Design review of the part built by this model. Coordinates are the model's own, in mm. Face numbers are marked on the shaded views. A direction names the side the tool comes from. Coordinates: 2 decimals unless noted, no trailing zeros. Order: outer loops, then holes, each group sorted by start corner. A loop starts at its lowest first (then second) coordinate and runs counter-clockwise, first axis right, second up. Notation, with made-up numbers: (31.25, -14) - (54.25, -14) arc R20 ccw to (54.25, 12) - close; hole circle Ø4 at (12, 62.25). An arc over 180 degrees is marked (long way). Write item = value, one per line. Start each with the question number.
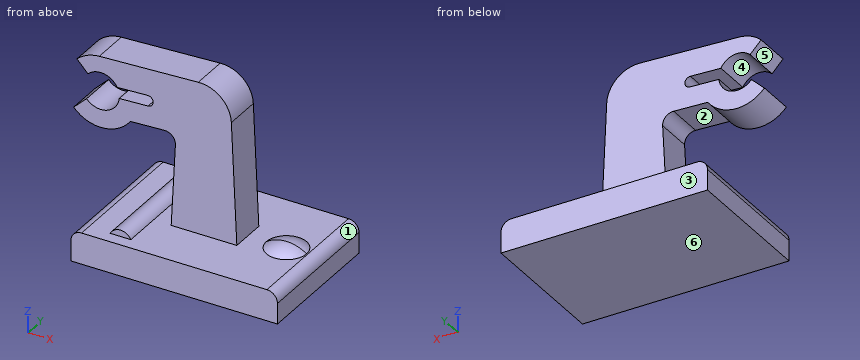
```python
from build123d import *

# Parameters (mm, degrees)
PAD_DEPTH        = 6.5
PAD001_DEPTH     = 5.35
REVOLUTION_ANGLE = -180
PAD002_DEPTH     = 1.75


with BuildPart() as part:
    # Sketch → Pad (new body)
    with BuildSketch(Plane.XZ):
        with BuildLine():
            Line((-9.75, 0), (9.75, 0))
            Line((9.75, 0), (9.75, 1.95))
            ThreePointArc((9.75, 1.95), (9.457107, 2.657107), (8.75, 2.95))
            Line((8.75, 2.95), (-8.75, 2.95))
            ThreePointArc((-8.75, 2.95), (-9.457107, 2.657107), (-9.75, 1.95))
            Line((-9.75, 1.95), (-9.75, 0))
        make_face()
    pad = extrude(amount=-PAD_DEPTH)

    # Sketch001 → Pad001 (join)
    with BuildSketch(Plane.XZ):
        with BuildLine():
            ThreePointArc((-4.775, 2.95), (-5.75, 3.55), (-6.725, 2.95))
            Line((-6.725, 2.95), (-4.775, 2.95))
        make_face()
    pad001 = extrude(amount=-PAD001_DEPTH)

    # Sketch002 → Revolution (revolve)
    with BuildSketch(Plane.XZ):
        with BuildLine():
            ThreePointArc((8.65, 2.95), (7.746243, 3.396436), (6.75, 3.55))
            Line((6.75, 3.55), (6.75, 0.241667))
            Line((8.65, 2.95), (6.75, 0.241667))
        make_face()
    revolution = revolve(axis=Axis((6.75, 0, 3.55), (0, 0, -1)), revolution_arc=REVOLUTION_ANGLE)

    # Sketch003 → Pad002 (join)
    with BuildSketch(Plane.XZ):
        with BuildLine():
            Line((-3.1, 2.95), (3.1, 2.95))
            Line((3.1, 2.95), (2.580696, 14.438223))
            ThreePointArc((2.580696, 14.438223), (1.609703, 16.515339), (-0.544721, 17.3))
            Line((-0.544721, 17.3), (-9.889288, 16.899445))
            ThreePointArc((-9.889288, 16.899445), (-11.025908, 16.641713), (-11.998693, 15.999824))
            Line((-11.998693, 15.999824), (-10.959931, 14.914345))
            ThreePointArc((-8.203688, 14.469402), (-9.471106, 15.377634), (-10.959931, 14.914345))
            Line((-8.203688, 14.469402), (-5.32558, 14.592772))
            ThreePointArc((-5.282715, 13.592772), (-4.804147, 14.114205), (-5.32558, 14.592772))
            Line((-5.282715, 13.592772), (-8.008679, 13.475924))
            ThreePointArc((-11.081461, 12.514345), (-9.227358, 11.979867), (-8.008679, 13.475924))
            Line((-12.311103, 11.337624), (-11.081461, 12.514345))
            ThreePointArc((-12.311103, 11.337624), (-9.56498, 10.204409), (-6.956, 11.62518))
            Line((-3.742396, 11.762931), (-6.956, 11.62518))
            ThreePointArc((-2.700889, 10.712502), (-2.989454, 11.467933), (-3.742396, 11.762931))
            Line((-3.1, 2.95), (-2.700889, 10.712502))
        make_face()
    pad002 = extrude(amount=-PAD002_DEPTH)

    # Mirrored: Pad, Pad001, Revolution, Pad002 across XZ
    add(pad.mirror(Plane.XZ))
    add(pad001.mirror(Plane.XZ))
    add(revolution.mirror(Plane.XZ))
    add(pad002.mirror(Plane.XZ))


solid = part.part
```
Item 1: Add section C-C on z = 1. Give the boundary of the cut face in (x, y).
Item 2: Add section B-B on x = -1.5. Give the boundary of the cut face in (y, z).
Item 3: For line 1 (Z direction, x = -8.25, y = 1.5); line 2 (X direction, y = -3.25, z = 2); line 3 (Z direction, x = -4, y = -3), list the stretches that pass through material, from the lowest coordinate up.
Item 4: Add section D-D on x = 3.75. Give the boundary of the cut face in (y, z).
Item 5: For the marked faces 4, 5 and 6, list the 3-axis set-ups (+Z, -Z, +X, -X, +Y, -Y) from which the entire face can be reached by the end or side of a thin tool; tool diameter is ignored.
Item 6: Mouldability with a two-part tool opening along X and no side actions: class the marked faces 1, 2 and 3 as +X half, -X half, draft (parallel to the pull), parting line (faces both ways), or undercut.
Item 7: Add section A-A on y = 3.25. Give the boundary of the cut face in (x, z) (3 decimals), plus the area to 3 significant figures.
Item 8: For P1, Ø6, axis at x = -3.5, y = -1, coming from the +Z side; P2, Ø5, axis at x = -4.5, z = 15.5, coming from the +Y side; P3, Ø4, axis at y = -3.5, z = 5, coming from the -X side; P4, Ø1, axis at y = -1, z = 1, coming from the -X side, all flat-tipped, find the tip position at first contact; note any pin that passes through.
Worked out:
q1.outline = (-9.75, -6.5) - (9.75, -6.5) - (9.75, 6.5) - (-9.75, 6.5) - close
q2.outline = (-6.5, 0) - (6.5, 0) - (6.5, 2.95) - (1.75, 2.95) - (1.75, 17.26) - (-1.75, 17.26) - (-1.75, 2.95) - (-6.5, 2.95) - close
q3.line_1 = 0 to 2.95, 10.54 to 12.75, 14.55 to 16.97
q3.line_2 = -9.75 to 9.75
q3.line_3 = 0 to 2.95
q4.outline = (-6.5, 0) - (6.5, 0) - (6.5, 2.95) - (-6.5, 2.95) - close
q5.face_4 = +Y, -Y
q5.face_5 = -X, +Y, -Y
q5.face_6 = -Z, +X, -X, +Y, -Y
q6.face_1 = +X half
q6.face_2 = undercut
q6.face_3 = draft
q7.outline = (-9.75, 0) - (9.75, 0) - (9.75, 1.95) arc R1 ccw to (8.75, 2.95) - (-4.775, 2.95) arc R1.092 ccw to (-6.725, 2.95) - (-8.75, 2.95) arc R1 ccw to (-9.75, 1.95) - close
q7.area = 57.9 mm2
q8.P1 = 17.3
q8.P2 = 1.75
q8.P3 = -6.7
q8.P4 = -9.75
